Check sheet for the drawn part. Datum: minimum x, y, z corner. Units: mm. Round coordinates to 2 decimals unless told otherwise and drop trailing zeros. Write each loop counter-clockwise with the first axis right and the second up, starting at its lowest first coordinate (ties: lowest second). Pieces come first, ordered by that corner, then holes. Notation, with made-up numbers: M 36.5,-34 L 89.5,-34 A34 ccw 89.5,-4 Z; hole C 28.25,36 d11. An arc over 180 degrees is marked long. One line per item, written item: value. Start each with the question number.
Item 1: Section check D-D, the plane z = 0.4. State how many separate pieces and enclosed holes the cut face has, then the cut area to 3 significant figures.
Item 2: Thickness scan on probe 1 along X at (y, z) = (7.62, 0.4); probe 2 along Y at (x, z) = (35, 0.3); probe 3 along X at (y, z) = (17.5, 0.65) (1 decimal). Record the ranges inside material, lowest first. Write a range as from..to.
Item 3: Section check B-B, the plane y = 19.05. Record the cut outline in (x, z).
Item 4: Section check A-A, the plane x = 19.05. Record the cut outline in (y, z).
Item 5: Section check C-C, the plane y = 7.62. Record the cut outline in (x, z).
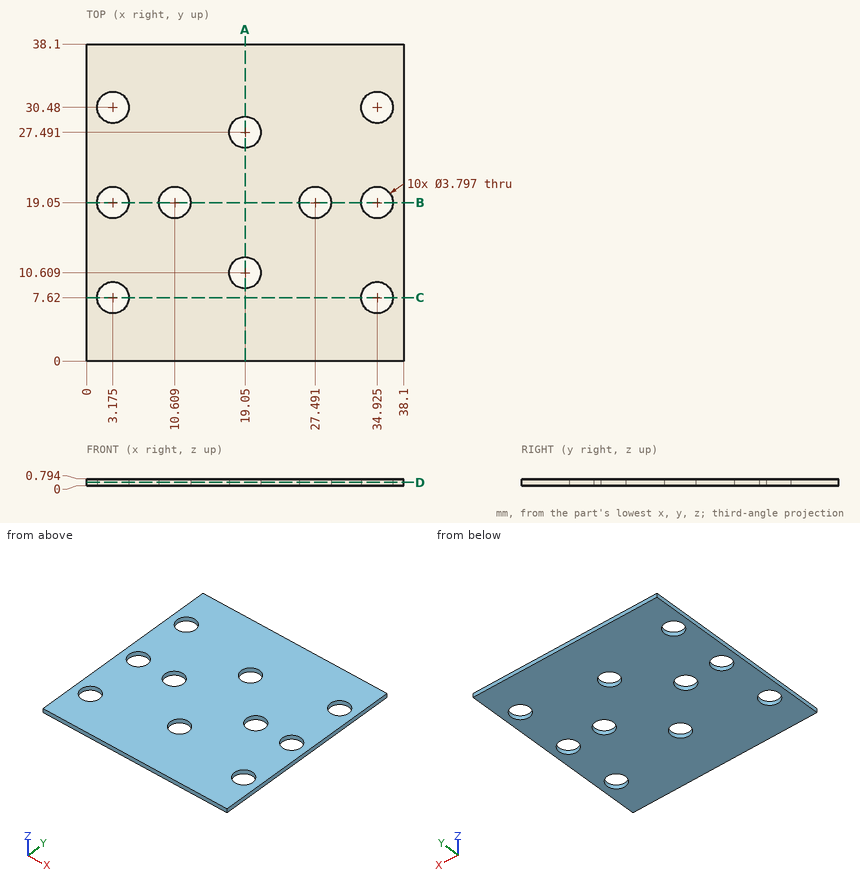
Response values:
1. separate pieces: 1
1. enclosed holes: 10
1. area: 1,340 mm2
2. probe 1: x = 0..1.28, 5.07..33.03, 36.82..38.1
2. probe 2: y = 0..5.72, 9.52..17.15, 20.95..28.58, 32.38..38.1
2. probe 3: x = 0..2.1, 4.3..9.5, 11.7..26.4, 28.6..33.8, 36..38.1
3. outline: M 0,0 L 1.28,0 L 1.28,0.79 L 0,0.79 Z; M 5.07,0 L 8.71,0 L 8.71,0.79 L 5.07,0.79 Z; M 12.51,0 L 25.59,0 L 25.59,0.79 L 12.51,0.79 Z; M 29.39,0 L 33.03,0 L 33.03,0.79 L 29.39,0.79 Z; M 36.82,0 L 38.1,0 L 38.1,0.79 L 36.82,0.79 Z
4. outline: M 0,0 L 8.71,0 L 8.71,0.79 L 0,0.79 Z; M 12.51,0 L 25.59,0 L 25.59,0.79 L 12.51,0.79 Z; M 29.39,0 L 38.1,0 L 38.1,0.79 L 29.39,0.79 Z
5. outline: M 0,0 L 1.28,0 L 1.28,0.79 L 0,0.79 Z; M 5.07,0 L 33.03,0 L 33.03,0.79 L 5.07,0.79 Z; M 36.82,0 L 38.1,0 L 38.1,0.79 L 36.82,0.79 Z
